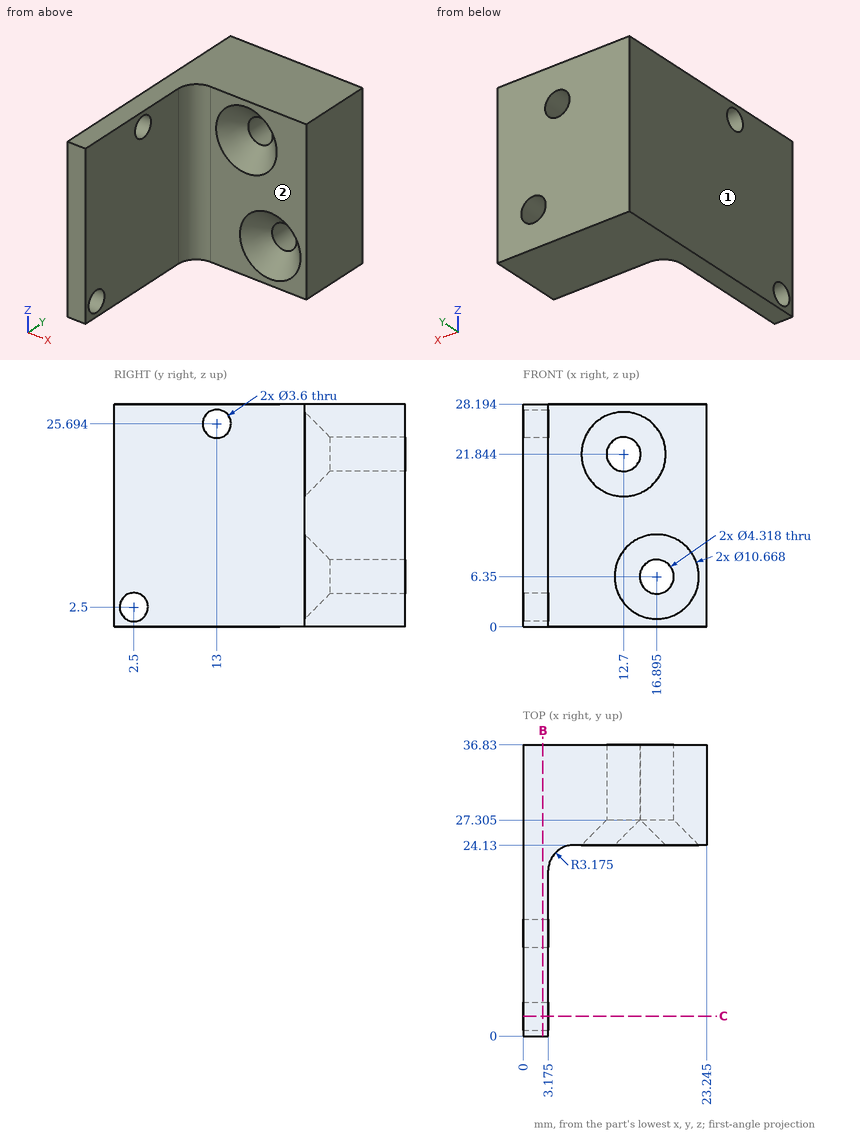
Answer from the drawing. Dimensions are ordinates in mm from the lowest x, y and z of the part. A direction names the side the tool comes from. Coordinates: 2 decimals unless noted, no trailing zeros. Write each loop counter-clockwise with the first axis right and the second up, starting at its lowest first coordinate (ties: lowest second). Pieces come first, ordered by that corner, then holes. Notation, with made-up numbers: M 21,26 L 62,26 A18 ccw 62,31 Z; hole C 62.5,-26.75 d11. An arc over 180 degrees is marked long. Write item = value, one per line.
1. For the marked faces 1 and 2, determine the directions among +Z, -Z, +X, -X, +Y, -Y from which every point of the face is accessible in a straight line to the end or side of a thin tool.
Solution:
face_1 = +Z, -Z, -X, +Y, -Y
face_2 = +Z, -Z, +X, -Y
2. The part is cut by section C-C (y = 2.5). Determine the outline of the cut face in (x, z) (1 decimal).
Solution:
outline = M 0,0 L 3.2,0 L 3.2,0.7 L 0,0.7 Z; M 0,4.3 L 3.2,4.3 L 3.2,28.2 L 0,28.2 Z
3. The part is cut by section B-B (x = 2.5). Determine the outline of the cut face in (y, z) (1 decimal).
Solution:
outline = M 0,0 L 36.8,0 L 36.8,28.2 L 0,28.2 Z; hole C 2.5,2.5 d3.6; hole C 13,25.7 d3.6
4. Straight lines are drawn through the part: line 1 (X direction, y = 13, z = 12) (1 decimal); line 2 (Y direction, x = 20.5, z = 13); line 3 (Z direction, x = 14, y = 33.5) (1 decimal). For each, find the intervals that lie inside material, in ascending order. Write a range as from..to.
Solution:
line_1 = 0..3.2
line_2 = 24.13..36.83
line_3 = 0..20.1, 23.6..28.2
5. Flat-ended cylindrical pins translate along their axes: pin 1 (3 mm diameter, centred on x = 20, z = 23, fed in from -Y); pin 2 (2 mm diameter, centred on y = 2.5, z = 2.5, fed in from -X); pin 3 (5 mm diameter, centred on x = 12.7, z = 21.844, fed in from -Y) (1 decimal); pin 4 (10.5 mm diameter, centred on y = 15.5, z = 10.5, fed in from +X) (1 decimal). Find the tip coordinate at first contact, or state that the pin passes through.
Solution:
pin_1 = 24.13
pin_2 = through
pin_3 = 27
pin_4 = 3.2
